Job drawing, mm, ordinate dimensions from the low corner. One solid piece. A direction names the side the tool comes from. Round coordinates to 2 decimals unless told otherwise and drop trailing zeros. Loops run counter-clockwise (first coordinate to the right, second up) from the corner with the lowest first, then second, coordinate; pieces in that order, holes last. Notation, with made-up numbers: M -34.75,23 L -17.75,23 A10 ccw -17.75,42 Z; hole C 76.25,21.5 d6. An arc over 180 degrees is marked long. Use a Markdown table: item, result. Add a question column.
(1) Band-saw the part on B-B, the plane z = 37. Write the cut outline in (x, y), and give its area (3 significant figures).
(2) Which spindle directions (+Z, -Z, +X, -X, +Y, -Y) get a long thin tool onto all of the face, cutting with end or side? Do the marked faces 1, 2, 3 and 4. Say none if no direction does.
(3) Wall check: L1, parallel to X at y = 11.15, z = 37; L2, parallel to Z at x = 9.5, y = 5.75; L3, parallel to Z at x = 3.7, y = 10.95. Give the ranges that are in metal, low to high.
(4) Band-saw the part on D-D, the plane z = 15.5. Write the cut outline in (x, y).
(5) Flat gauge pins, fed straight in: P1, Ø2.5, axis at x = 3.7, z = 37, coming from the +Y side; P2, Ø5, axis at y = 5, z = 7.5, coming from the +X side; P3, Ø1.5, axis at x = 14.5, y = 8, coming from the -Z side; P4, Ø10, axis at x = 5, z = 8, coming from the +Y side. Where does each tip first touch, or does it go through?
(6) Band-saw the part on A-A, the plane y = 5.5. Write the cut outline in (x, z).
(7) Band-saw the part on C-C, the plane x = 6. Write the cut outline in (y, z).
(8) Two-plate mould, pull along X, no slides. Class the marked faces 5, 6 and 7: released by +X, released by -X, zero draft, split by the parting line, or undercut.
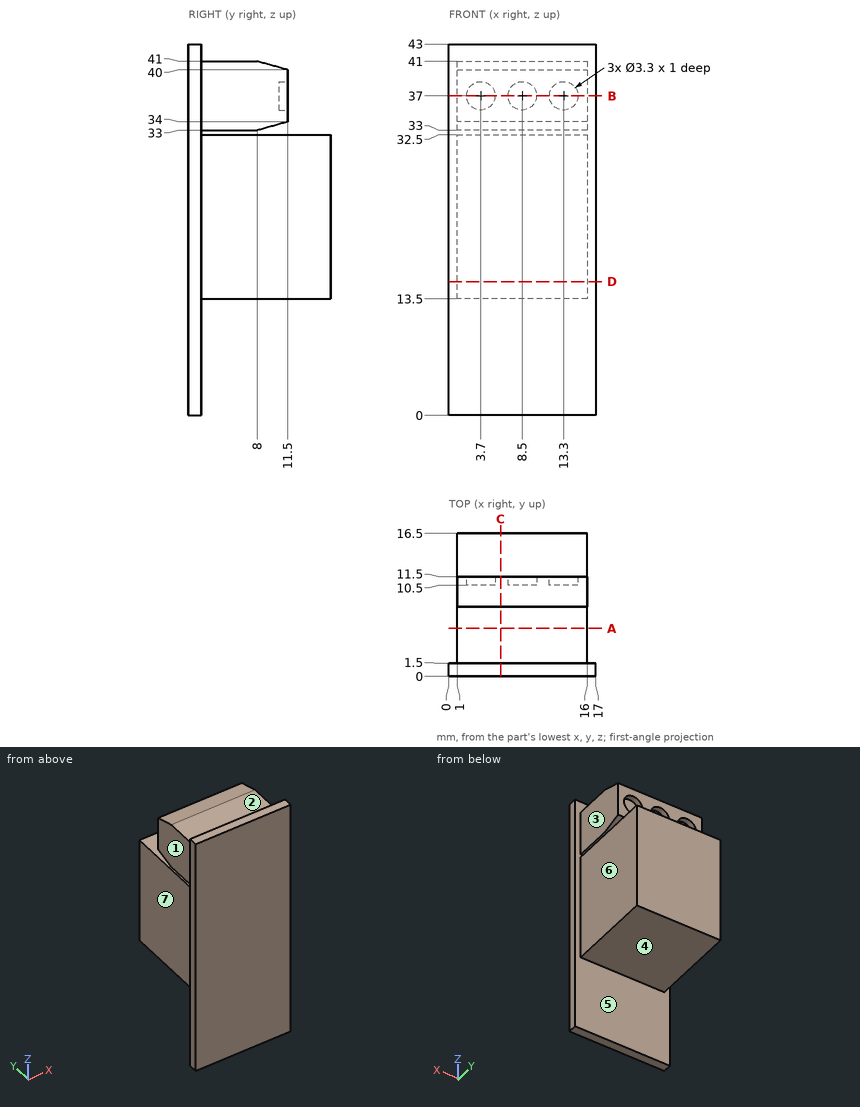
Return value:
| question | item | result |
|---|---|---|
| 1 | outline | M 0,0 L 17,0 L 17,1.5 L 16,1.5 L 16,11.5 L 14.95,11.5 L 14.95,10.5 L 11.65,10.5 L 11.65,11.5 L 10.15,11.5 L 10.15,10.5 L 6.85,10.5 L 6.85,11.5 L 5.35,11.5 L 5.35,10.5 L 2.05,10.5 L 2.05,11.5 L 1,11.5 L 1,1.5 L 0,1.5 Z |
| 1 | area | 166 mm^2 |
| 2 | face 1 | +Z, -Z, -X, +Y |
| 2 | face 2 | +Z, +X, -X, +Y |
| 2 | face 3 | +Z, -Z, +X, +Y |
| 2 | face 4 | -Z, +X, -X, +Y |
| 3 | L1 | 1 to 2.05, 5.35 to 6.85, 10.15 to 11.65, 14.95 to 16 |
| 3 | L2 | 13.5 to 32.5, 33 to 41 |
| 3 | L3 | 13.5 to 32.5, 33.84 to 35.35, 38.65 to 40.16 |
| 4 | outline | M 0,0 L 17,0 L 17,1.5 L 16,1.5 L 16,16.5 L 1,16.5 L 1,1.5 L 0,1.5 Z |
| 5 | P1 | y = 10.5 |
| 5 | P2 | through |
| 5 | P3 | z = 13.5 |
| 5 | P4 | y = 1.5 |
| 6 | outline | M 1,13.5 L 16,13.5 L 16,32.5 L 1,32.5 Z; M 1,33 L 16,33 L 16,41 L 1,41 Z |
| 7 | outline | M 0,0 L 1.5,0 L 1.5,13.5 L 16.5,13.5 L 16.5,32.5 L 1.5,32.5 L 1.5,33 L 8,33 L 11.5,34 L 11.5,40 L 8,41 L 1.5,41 L 1.5,43 L 0,43 Z |
| 8 | face 5 | zero draft |
| 8 | face 6 | released by +X |
| 8 | face 7 | released by -X |
